The drawing under review shows one solid part. Ordinate dimensions are in mm from its lowest x, y, z. A direction names the side the tool comes from. Coordinates: 2 decimals unless noted, no trailing zeros. Loops run counter-clockwise (first coordinate to the right, second up) from the corner with the lowest first, then second, coordinate; pieces in that order, holes last. Notation, with made-up numbers: M 88.25,72 L 108.25,72 A24 ccw 108.25,104 Z; hole C 33,33.5 d5. An arc over 180 degrees is marked long. Answer as CSV lines item,"result". Start each with the question number.
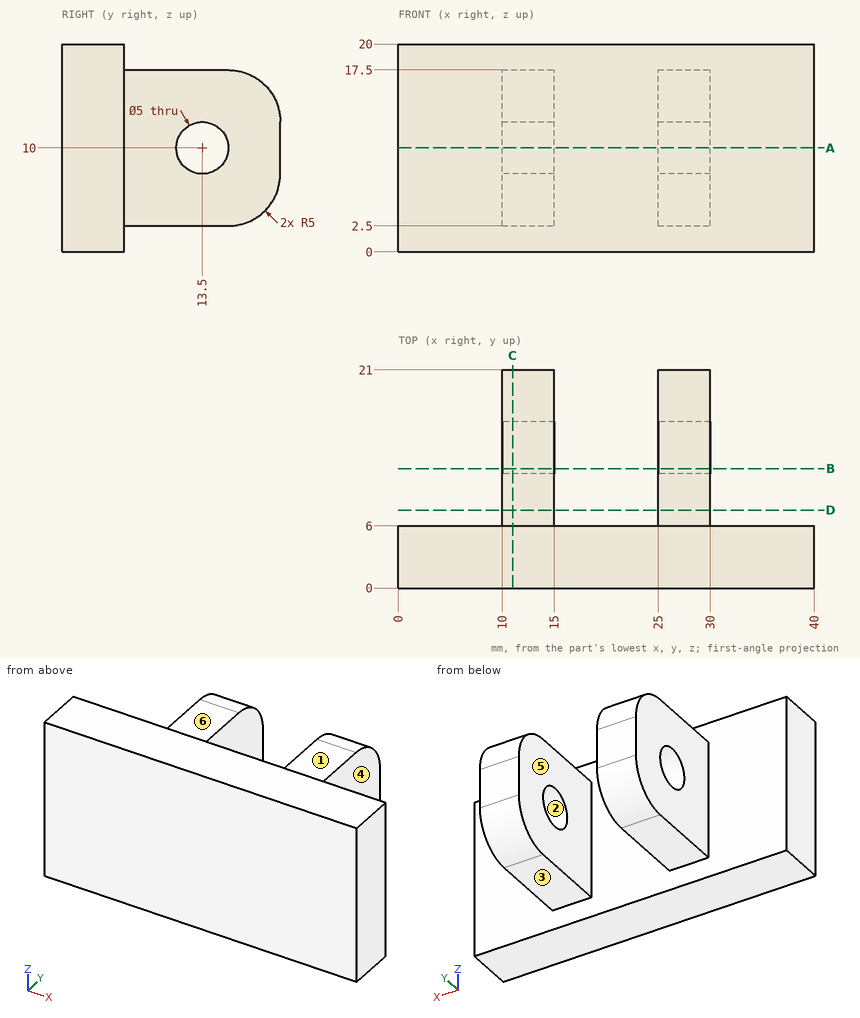
Item 1: Add section D-D (y = 7.5). Give the boundary of the cut face in (x, z), plus the area to 3 significant figures.
Item 2: For line 1 along X through (y, z) = (14.5, 15.25); line 2 along Y through (x, z) = (27.15, 10); line 3 along Y through (x, z) = (3, 7.25), list the stretches that pass through material, from the lowest coordinate up. Write a range as from..to.
Item 3: Add section B-B (y = 11.5). Give the boundary of the cut face in (x, z).
Item 4: For the marked faces 1, 2 and 3, list the 3-axis set-ups (+Z, -Z, +X, -X, +Y, -Y) from which the entire face can be reached by the end or side of a thin tool; tool diameter is ignored.
Item 5: Add section A-A (z = 10). Give the boundary of the cut face in (x, y), plus the area to 3 significant figures.
Item 6: Mouldability with a two-part tool opening along X and no side actions: class the marked faces 4, 5 and 6 as released by +X, released by -X, zero draft, split by the parting line, or undercut.
Item 7: For pin 1 (6 mm diameter, centred on y = 13.5, z = 10, fed in from -X); pin 2 (2.5 mm diameter, centred on x = 12, y = 10.5, fed in from -Z); pin 3 (5 mm diameter, centred on x = 23.5, z = 3, fed in from +Y); pin 4 (5 mm diameter, centred on x = 22, y = 15, fed in from +Z), all flat-tipped, find the tip position at first contact; note any pin that passes through.
Item 8: Add section C-C (x = 11). Give the boundary of the cut face in (y, z).
Response:
1,outline,"M 10,2.5 L 15,2.5 L 15,17.5 L 10,17.5 Z; M 25,2.5 L 30,2.5 L 30,17.5 L 25,17.5 Z"
1,area,"150 mm²"
2,line 1,"10..15, 25..30"
2,line 2,"0..11, 16..21"
2,line 3,"0..6"
3,outline,"M 10,2.5 L 15,2.5 L 15,8.5 L 10,8.5 Z; M 10,11.5 L 15,11.5 L 15,17.5 L 10,17.5 Z; M 25,2.5 L 30,2.5 L 30,8.5 L 25,8.5 Z; M 25,11.5 L 30,11.5 L 30,17.5 L 25,17.5 Z"
4,face 1,"+Z, +X, -X, +Y"
4,face 2,"+X, -X"
4,face 3,"-Z, +X, -X, +Y"
5,outline,"M 0,0 L 40,0 L 40,6 L 30,6 L 30,11 L 25,11 L 25,6 L 15,6 L 15,11 L 10,11 L 10,6 L 0,6 Z; M 10,16 L 15,16 L 15,21 L 10,21 Z; M 25,16 L 30,16 L 30,21 L 25,21 Z"
5,area,"340 mm²"
6,face 4,"released by +X"
6,face 5,"undercut"
6,face 6,"zero draft"
7,pin 1,"x = 10"
7,pin 2,"z = 2.5"
7,pin 3,"y = 20.33"
7,pin 4,"through"
8,outline,"M 0,0 L 6,0 L 6,2.5 L 16,2.5 A5 ccw 21,7.5 L 21,12.5 A5 ccw 16,17.5 L 6,17.5 L 6,20 L 0,20 Z; hole C 13.5,10 d5"
